from build123d import *

# Parameters (mm, degrees)
SKETCH1_W                                         = 152.4
SKETCH1_H                                         = 101.6
BOSS_EXTRUDE1_DEPTH                               = 3.81
SKETCH2_W                                         = 152.4
SKETCH2_H                                         = 101.6
SKETCH2_W_2                                       = 147.32
SKETCH2_H_2                                       = 96.52
BOSS_EXTRUDE2_DEPTH                               = 44.45
BOSS_EXTRUDE3_DEPTH                               = 44.45
CUT_EXTRUDE1_START                                = 28.575
SKETCH3_3_R                                       = 1.27
CUT_EXTRUDE1_DEPTH                                = 15.875
MIRROR2_COPY_1_DEPTH                              = 44.45
MIRROR2_START                                     = 28.575
MIRROR2_COPY_2_SKETCH_R                           = 1.27
MIRROR2_COPY_2_DEPTH                              = 15.875
CUT_EXTRUDE2_REACH                                = 191.413
SKETCH6_R                                         = 5.5
SKETCH6_W                                         = 27.686
SKETCH6_H                                         = 47.244
SKETCH7_W                                         = 1.016
SKETCH7_H                                         = 47.244
CUT_EXTRUDE3_DEPTH                                = 39.243
SKETCH8_R                                         = 1.651
BOSS_EXTRUDE4_DEPTH                               = 3.81
FILLET1_R                                         = 1.5875
FILLET1_OF_MIRROR5_R                              = 1.5875
CUT_EXTRUDE4_REACH                                = 196.906
LPATTERN1_COUNT                                   = 9
LPATTERN1_PITCH                                   = 10.16
CSK_FOR_M3_FLAT_HEAD_MACHINE_SCREW1_D             = 3.4
CSK_FOR_M3_FLAT_HEAD_MACHINE_SCREW1_DEPTH         = 6.35
CSK_FOR_M3_FLAT_HEAD_MACHINE_SCREW1_CSINK_D       = 6.3
CSK_FOR_M3_FLAT_HEAD_MACHINE_SCREW1_CSINK_ANGLE   = 90
CSK_FOR_M3_FLAT_HEAD_MACHINE_SCREW1_TIP           = 1.021463052
CSK_FOR_M3_FLAT_HEAD_MACHINE_SCREW2_D             = 3.4
CSK_FOR_M3_FLAT_HEAD_MACHINE_SCREW2_DEPTH         = 6.35
CSK_FOR_M3_FLAT_HEAD_MACHINE_SCREW2_CSINK_D       = 6.3
CSK_FOR_M3_FLAT_HEAD_MACHINE_SCREW2_CSINK_ANGLE   = 90
CSK_FOR_M3_FLAT_HEAD_MACHINE_SCREW2_TIP           = 1.021463052
CSK_FOR_4_FLAT_HEAD_MACHINE_SCREW_100_D           = 3.2639
CSK_FOR_4_FLAT_HEAD_MACHINE_SCREW_100_DEPTH       = 6.35
CSK_FOR_4_FLAT_HEAD_MACHINE_SCREW_100_CSINK_D     = 5.715
CSK_FOR_4_FLAT_HEAD_MACHINE_SCREW_100_CSINK_ANGLE = 100
CSK_FOR_4_FLAT_HEAD_MACHINE_SCREW_100_TIP         = 0.980574487
CSK_FOR_4_FLAT_HEAD_MACHINE_SCREW_2_D             = 3.2639
CSK_FOR_4_FLAT_HEAD_MACHINE_SCREW_2_DEPTH         = 6.35
CSK_FOR_4_FLAT_HEAD_MACHINE_SCREW_2_CSINK_D       = 5.715
CSK_FOR_4_FLAT_HEAD_MACHINE_SCREW_2_CSINK_ANGLE   = 100
CSK_FOR_4_FLAT_HEAD_MACHINE_SCREW_2_TIP           = 0.980574487


with BuildPart() as part:
    # Sketch1 → Boss-Extrude1 (new body)
    with BuildSketch(Plane.XY):
        with Locations((76.2, 50.8)):
            Rectangle(SKETCH1_W, SKETCH1_H)
    extrude(amount=BOSS_EXTRUDE1_DEPTH)

    # Sketch2 → Boss-Extrude2 (add)
    with BuildSketch(Plane.XY.offset(3.81)):
        with Locations((76.2, 50.8)):
            Rectangle(SKETCH2_W, SKETCH2_H)
        with Locations((76.2, 50.8)):
            Rectangle(SKETCH2_W_2, SKETCH2_H_2, mode=Mode.SUBTRACT)
    extrude(amount=BOSS_EXTRUDE2_DEPTH)

    # Sketch3 → Boss-Extrude3 (add)
    with BuildSketch(Plane.XY.offset(3.81)):
        Polygon((137.16, 99.06), (149.86, 86.36), (149.86, 99.06), align=None)
    boss_extrude3 = extrude(amount=BOSS_EXTRUDE3_DEPTH)

    # Sketch3<3> → Cut-Extrude1 (cut)
    with BuildSketch(Plane.XY.offset(3.81).offset(CUT_EXTRUDE1_START)):
        with Locations((146.05, 95.25)):
            Circle(SKETCH3_3_R)
    cut_extrude1 = extrude(amount=CUT_EXTRUDE1_DEPTH, mode=Mode.SUBTRACT)

    # Mirror1: Boss-Extrude3, Cut-Extrude1 across plane
    add(boss_extrude3.mirror(Plane(origin=(76.2, 0, 0), x_dir=(0, 0, 1), z_dir=(1, 0, 0))))
    add(cut_extrude1.mirror(Plane(origin=(76.2, 0, 0), x_dir=(0, 0, 1), z_dir=(1, 0, 0))), mode=Mode.SUBTRACT)

    # Mirror2: Boss-Extrude3, Cut-Extrude1 across plane
    add(boss_extrude3.mirror(Plane(origin=(0, 50.8, 0), x_dir=(0, 0, 1), z_dir=(0, -1, 0))))
    add(cut_extrude1.mirror(Plane(origin=(0, 50.8, 0), x_dir=(0, 0, 1), z_dir=(0, -1, 0))), mode=Mode.SUBTRACT)

    # Mirror2 copy 1 sketch → Mirror2 copy 1 (add)
    with BuildSketch(Plane(origin=(152.4, 101.6, 3.81), x_dir=(-1, 0, 0), z_dir=(0, 0, 1))):
        Polygon((137.16, 99.06), (149.86, 86.36), (149.86, 99.06), align=None)
    extrude(amount=MIRROR2_COPY_1_DEPTH)

    # Mirror2 copy 2 sketch → Mirror2 copy 2 (cut)
    with BuildSketch(Plane(origin=(152.4, 101.6, 3.81), x_dir=(-1, 0, 0), z_dir=(0, 0, 1)).offset(MIRROR2_START)):
        with Locations((146.05, 95.25)):
            Circle(MIRROR2_COPY_2_SKETCH_R)
    extrude(amount=MIRROR2_COPY_2_DEPTH, mode=Mode.SUBTRACT)

    # Sketch6 → Cut-Extrude2 (cut, up to next)
    with BuildSketch(Plane.ZY, mode=Mode.PRIVATE) as cut_extrude2_sk1:
        with Locations((24.13, 25.4)):
            Circle(SKETCH6_R)
    cut_extrude2_tool1 = extrude(cut_extrude2_sk1.sketch, amount=-CUT_EXTRUDE2_REACH, mode=Mode.PRIVATE) & part.part
    # Sketch6 → Cut-Extrude2 (cut, up to next)
    with BuildSketch(Plane.ZY, mode=Mode.PRIVATE) as cut_extrude2_sk2:
        with Locations((24.13, 62.738)):
            Rectangle(SKETCH6_W, SKETCH6_H)
    cut_extrude2_tool2 = extrude(cut_extrude2_sk2.sketch, amount=-CUT_EXTRUDE2_REACH, mode=Mode.PRIVATE) & part.part
    add(cut_extrude2_tool1.solids().sort_by_distance((0, 25.4, 24.13))[0], mode=Mode.SUBTRACT)
    add(cut_extrude2_tool2.solids().sort_by_distance((0, 62.738, 24.13))[0], mode=Mode.SUBTRACT)

    # Sketch7 → Cut-Extrude3 (cut)
    with BuildSketch(Plane.XY.offset(48.26)):
        with Locations((2.032, 62.738)):
            Rectangle(SKETCH7_W, SKETCH7_H)
    extrude(amount=-CUT_EXTRUDE3_DEPTH, mode=Mode.SUBTRACT)

    # Sketch8 → Boss-Extrude4 (add)
    # profile 1 of 2: a face of its own
    with BuildSketch(Plane(origin=(0, 0, 0), x_dir=(-1, 0, 0), z_dir=(0, 0, -1))):
        with BuildLine():
            Line((-144.526, 106.68), (-144.526, 101.6))
            Line((-144.526, 101.6), (-134.874, 101.6))
            Line((-134.874, 101.6), (-134.874, 106.68))
            ThreePointArc((-134.874, 106.68), (-139.7, 111.506), (-144.526, 106.68))
        make_face()
        with Locations((-139.7, 106.68)):
            Circle(SKETCH8_R, mode=Mode.SUBTRACT)
    # profile 2 of 2: a face of its own
    with BuildSketch(Plane(origin=(0, 0, 0), x_dir=(-1, 0, 0), z_dir=(0, 0, -1))):
        with BuildLine():
            Line((-134.874, 0), (-134.874, -5.08))
            ThreePointArc((-134.874, -5.08), (-139.7, -9.906), (-144.526, -5.08))
            Line((-144.526, -5.08), (-144.526, 0))
            Line((-144.526, 0), (-134.874, 0))
        make_face()
        with Locations((-139.7, -5.08)):
            Circle(SKETCH8_R, mode=Mode.SUBTRACT)
    boss_extrude4 = extrude(amount=-BOSS_EXTRUDE4_DEPTH)

    # Fillet1
    fillet1_edges = [part.edges().sort_by_distance(p)[0] for p in [
        (139.7, 101.6, 3.81),
        (134.874, 101.6, 1.905),
        (144.526, 101.6, 1.905),
        (139.7, 0, 3.81),
        (144.526, 0, 1.905),
        (134.874, 0, 1.905),
    ]]
    fillet(fillet1_edges, radius=FILLET1_R)

    # Mirror5: Boss-Extrude4 across plane
    add(boss_extrude4.mirror(Plane(origin=(76.2, 0, 0), x_dir=(0, 0, 1), z_dir=(1, 0, 0))))

    # Fillet1 of Mirror5
    fillet1_of_mirror5_edges = [part.edges().sort_by_distance(p)[0] for p in [
        (12.7, 101.6, 3.81),
        (17.526, 101.6, 1.905),
        (7.874, 101.6, 1.905),
        (12.7, 0, 3.81),
        (7.874, 0, 1.905),
        (17.526, 0, 1.905),
    ]]
    fillet(fillet1_of_mirror5_edges, radius=FILLET1_OF_MIRROR5_R)

    # Sketch9 → Cut-Extrude4 (cut, up to next)
    with BuildSketch(Plane.XZ, mode=Mode.PRIVATE) as cut_extrude4_sk1:
        with BuildLine():
            Line((39.37, 33.655), (39.37, 14.605))
            ThreePointArc((39.37, 14.605), (38.1, 13.335), (36.83, 14.605))
            Line((36.83, 14.605), (36.83, 33.655))
            ThreePointArc((36.83, 33.655), (38.1, 34.925), (39.37, 33.655))
        make_face()
    cut_extrude4_tool1 = extrude(cut_extrude4_sk1.sketch, amount=-CUT_EXTRUDE4_REACH, mode=Mode.PRIVATE) & part.part
    cut_extrude4 = cut_extrude4_tool1.solids().sort_by_distance((38.1, 0, 24.13))[0]
    add(cut_extrude4, mode=Mode.SUBTRACT)

    # LPattern1: Cut-Extrude4 ×9
    with Locations(*[(i * LPATTERN1_PITCH, 0, 0) for i in range(1, LPATTERN1_COUNT)]):
        add(cut_extrude4, mode=Mode.SUBTRACT)

    # CSK for M3 Flat Head Machine Screw1
    with Locations(Plane(origin=(0, 0, 0), x_dir=(-1, 0, 0), z_dir=(0, 0, -1))):
        with Locations((-70.0024, 74.6252), (-70.0024, 46.9392), (-105.8164, 46.9392)):
            CounterSinkHole(CSK_FOR_M3_FLAT_HEAD_MACHINE_SCREW1_D / 2, CSK_FOR_M3_FLAT_HEAD_MACHINE_SCREW1_CSINK_D / 2, depth=CSK_FOR_M3_FLAT_HEAD_MACHINE_SCREW1_DEPTH, counter_sink_angle=CSK_FOR_M3_FLAT_HEAD_MACHINE_SCREW1_CSINK_ANGLE)
            with Locations((0, 0, -(CSK_FOR_M3_FLAT_HEAD_MACHINE_SCREW1_DEPTH + CSK_FOR_M3_FLAT_HEAD_MACHINE_SCREW1_TIP / 2))):  # 118° drill point
                Cone(0, CSK_FOR_M3_FLAT_HEAD_MACHINE_SCREW1_D / 2, CSK_FOR_M3_FLAT_HEAD_MACHINE_SCREW1_TIP, mode=Mode.SUBTRACT)

    # CSK for M3 Flat Head Machine Screw2
    with Locations(Plane(origin=(0, 101.6, 0), x_dir=(1, 0, 0), z_dir=(0, 1, 0))):
        with Locations((39.751, -17.018), (127.2286, -22.987)):
            CounterSinkHole(CSK_FOR_M3_FLAT_HEAD_MACHINE_SCREW2_D / 2, CSK_FOR_M3_FLAT_HEAD_MACHINE_SCREW2_CSINK_D / 2, depth=CSK_FOR_M3_FLAT_HEAD_MACHINE_SCREW2_DEPTH, counter_sink_angle=CSK_FOR_M3_FLAT_HEAD_MACHINE_SCREW2_CSINK_ANGLE)
            with Locations((0, 0, -(CSK_FOR_M3_FLAT_HEAD_MACHINE_SCREW2_DEPTH + CSK_FOR_M3_FLAT_HEAD_MACHINE_SCREW2_TIP / 2))):  # 118° drill point
                Cone(0, CSK_FOR_M3_FLAT_HEAD_MACHINE_SCREW2_D / 2, CSK_FOR_M3_FLAT_HEAD_MACHINE_SCREW2_TIP, mode=Mode.SUBTRACT)

    # CSK for _4 Flat Head Machine Screw _100
    with Locations(Plane(origin=(0, 101.6, 0), x_dir=(1, 0, 0), z_dir=(0, 1, 0))):
        with Locations((30.6197, -32.3977), (132.2197, -32.3977)):
            CounterSinkHole(CSK_FOR_4_FLAT_HEAD_MACHINE_SCREW_100_D / 2, CSK_FOR_4_FLAT_HEAD_MACHINE_SCREW_100_CSINK_D / 2, depth=CSK_FOR_4_FLAT_HEAD_MACHINE_SCREW_100_DEPTH, counter_sink_angle=CSK_FOR_4_FLAT_HEAD_MACHINE_SCREW_100_CSINK_ANGLE)
            with Locations((0, 0, -(CSK_FOR_4_FLAT_HEAD_MACHINE_SCREW_100_DEPTH + CSK_FOR_4_FLAT_HEAD_MACHINE_SCREW_100_TIP / 2))):  # 118° drill point
                Cone(0, CSK_FOR_4_FLAT_HEAD_MACHINE_SCREW_100_D / 2, CSK_FOR_4_FLAT_HEAD_MACHINE_SCREW_100_TIP, mode=Mode.SUBTRACT)

    # CSK for _4 Flat Head Machine Screw _ 2
    with Locations(Plane(origin=(0, 0, 0), x_dir=(-1, 0, 0), z_dir=(0, 0, -1))):
        with Locations((-29.9085, 26.2255), (-132.3721, 93.3323)):
            CounterSinkHole(CSK_FOR_4_FLAT_HEAD_MACHINE_SCREW_2_D / 2, CSK_FOR_4_FLAT_HEAD_MACHINE_SCREW_2_CSINK_D / 2, depth=CSK_FOR_4_FLAT_HEAD_MACHINE_SCREW_2_DEPTH, counter_sink_angle=CSK_FOR_4_FLAT_HEAD_MACHINE_SCREW_2_CSINK_ANGLE)
            with Locations((0, 0, -(CSK_FOR_4_FLAT_HEAD_MACHINE_SCREW_2_DEPTH + CSK_FOR_4_FLAT_HEAD_MACHINE_SCREW_2_TIP / 2))):  # 118° drill point
                Cone(0, CSK_FOR_4_FLAT_HEAD_MACHINE_SCREW_2_D / 2, CSK_FOR_4_FLAT_HEAD_MACHINE_SCREW_2_TIP, mode=Mode.SUBTRACT)


solid = part.part
Here's how the part is built. I have some questions about the finished solid (model axes, mm). A direction names the side the tool comes from. Give positions to 0.01 mm unless a question says otherwise; leave off trailing zeros. Loops run counter-clockwise (first coordinate to the right, second up) from the corner with the lowest first, then second, coordinate; pieces in that order, holes last. Notation, with made-up numbers: (55, 67) -> (69, 67) arc R23 ccw to (69, 92) -> close; hole circle Ø2 at (11, -14). An arc over 180 degrees is marked (long way). One line per item, written item: value.
Q1. Suppose I cut it at B-B on y = 83.5. Please give me the cut outline in (x, z).
Answers follow:
outline: (0, 0) -> (152.4, 0) -> (152.4, 48.26) -> (149.86, 48.26) -> (149.86, 3.81) -> (2.54, 3.81) -> (2.54, 9.02) -> (1.52, 9.02) -> (1.52, 10.29) -> (0, 10.29) -> close; (0, 37.97) -> (1.52, 37.97) -> (1.52, 48.26) -> (0, 48.26) -> close
Q2. If I drill on line 1 along Y through (x, z) = (139.7, 1.05); line 2 along X through (y, z) = (16, 43); line 3 along Y through (x, z) = (65, 25), over which ranges is the centre line in solid material (lowest first)?
Answers follow:
line 1: -9.91 to -6.73, -3.43 to 105.03, 108.33 to 111.51
line 2: 0 to 2.54, 149.86 to 152.4
line 3: 0 to 2.54, 99.06 to 101.6
Q3. On a 3-axis mill with a long thin cutter (end or side, diameter ignored), from which of +Z, -Z, +X, -X, +Y, -Y can I reach the whole of each face in a straight line? I mean faces 1 (the face through (7.874, 105, 2)), 2 (the face through (7.874, -3, 2)), 3 (the face through (143.42, 8.8, 25.72)). Say none if no direction works.
Answers follow:
face 1: +Z, -Z, -X, +Y
face 2: +Z, -Z, -X, -Y
face 3: +Z
Q4. Suppose I cut it at D-D on x = 63. Please give me the cut outline in (y, z), then the cut area to 3 significant figures.
Answers follow:
outline: (0, 0) -> (101.6, 0) -> (101.6, 48.26) -> (99.06, 48.26) -> (99.06, 3.81) -> (2.54, 3.81) -> (2.54, 48.26) -> (0, 48.26) -> close
area: 613 mm^2
Q5. I'm going to push flat-ended pins straight in: pin 1 Ø5.5 at (x, y) = (70, 46.94) entering from +Z; pin 2 Ø2 at (x, y) = (146.5, 6) entering from +Z; pin 3 Ø2.5 at (x, z) = (132.22, 32.4) entering from +Y; pin 4 Ø10 at (x, z) = (22.5, 40) entering from +Y. Where does each tip first touch, or does it pass through?
Answers follow:
pin 1: z = 3.81
pin 2: z = 48.26
pin 3: y = 2.54
pin 4: y = 101.6
Q6. Suppose I cut it at C-C on z = 45. Please give me the cut outline in (x, y).
Answers follow:
outline: (0, 0) -> (152.4, 0) -> (152.4, 101.6) -> (0, 101.6) -> close; hole (1.52, 39.12) -> (2.54, 39.12) -> (2.54, 15.24) -> (15.24, 2.54) -> (137.16, 2.54) -> (149.86, 15.24) -> (149.86, 86.36) -> (137.16, 99.06) -> (15.24, 99.06) -> (2.54, 86.36) -> (1.52, 86.36) -> close; hole circle Ø2.54 at (6.35, 6.35); hole circle Ø2.54 at (6.35, 95.25); hole circle Ø2.54 at (146.05, 6.35); hole circle Ø2.54 at (146.05, 95.25)
Q7. We'd pull the mould along X, two halves only. Please class faces 4 (the face through (93.5, 99.5, 48.26)), 5 (the face through (144.526, -3, 2)), 6 (the face through (12.806, 111.505, 1.878)), 7 (the face through (17.526, -3, 2)): pulls with the +X half, pulls with the -X half, needs draft (parallel to the pull), parting line crosses it, or undercut.
Answers follow:
face 4: needs draft
face 5: pulls with the +X half
face 6: undercut
face 7: undercut
Q8. Suppose I cut it at A-A on x = 12.7. Please give me the cut outline in (y, z) (1 decimal), then the cut area to 3 significant figures.
Answers follow:
outline: (-9.9, 0) -> (-6.7, 0) -> (-6.7, 3.8) -> (-9.9, 3.8) -> close; (-3.4, 0) -> (105, 0) -> (105, 3.8) -> (103.2, 3.8) arc R1.6 cw to (101.6, 5.4) -> (101.6, 48.3) -> (96.5, 48.3) -> (96.5, 3.8) -> (5.1, 3.8) -> (5.1, 48.3) -> (0, 48.3) -> (0, 5.4) arc R1.6 cw to (-1.6, 3.8) -> (-3.4, 3.8) -> close; (108.3, 0) -> (111.5, 0) -> (111.5, 3.8) -> (108.3, 3.8) -> close
area: 890 mm^2
